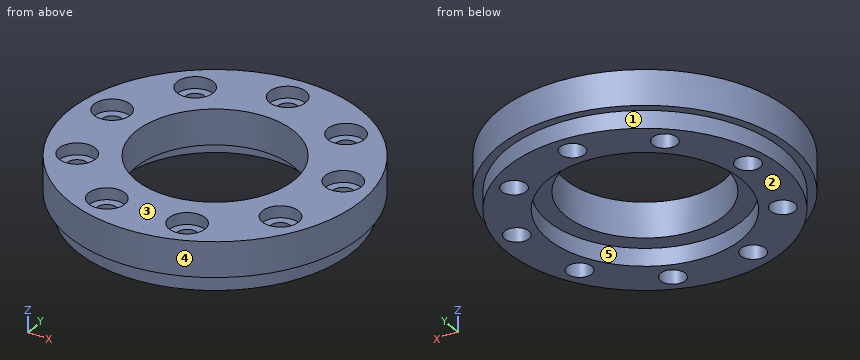
```python
from build123d import *

# Parameters (mm, degrees)
ESQUISSE1_R             = 24.95
BOSS_EXTRU_1_DEPTH      = 6
ESQUISSE3_R             = 3.1
ENL_V_MAT_EXTRU_1_DEPTH = 2
ESQUISSE4_R             = 1.7
ENL_V_MAT_EXTRU_2_DEPTH = 7
ESQUISSE5_R             = 23.5
ESQUISSE5_R_2           = 16.5
ESQUISSE5_R_3           = 1.7
BOSS_EXTRU_2_DEPTH      = 3
ESQUISSE6_R             = 2.1
ENL_V_MAT_EXTRU_3_DEPTH = 5.7
ESQUISSE7_R             = 13.5
ENL_V_MAT_EXTRU_4_DEPTH = 7


with BuildPart() as part:
    # Esquisse1 → Boss.-Extru.1 (new body)
    with BuildSketch(Plane.XY):
        Circle(ESQUISSE1_R)
    extrude(amount=BOSS_EXTRU_1_DEPTH)

    # Esquisse3 → Enlèv. mat.-Extru.1 (cut)
    with BuildSketch(Plane(origin=(0, 0, 6), x_dir=(-1, 0, 0), z_dir=(0, 0, -1))):
        with Locations((0, 20)):
            Circle(ESQUISSE3_R)
        with Locations((12.855752194, 15.320888862)):
            Circle(ESQUISSE3_R)
        with Locations((19.69615506, 3.472963553)):
            Circle(ESQUISSE3_R)
        with Locations((17.320508076, -10)):
            Circle(ESQUISSE3_R)
        with Locations((6.840402867, -18.793852416)):
            Circle(ESQUISSE3_R)
        with Locations((-6.840402867, -18.793852416)):
            Circle(ESQUISSE3_R)
        with Locations((-17.320508076, -10)):
            Circle(ESQUISSE3_R)
        with Locations((-19.69615506, 3.472963553)):
            Circle(ESQUISSE3_R)
        with Locations((-12.855752194, 15.320888862)):
            Circle(ESQUISSE3_R)
    extrude(amount=ENL_V_MAT_EXTRU_1_DEPTH, mode=Mode.SUBTRACT)

    # Esquisse4 → Enlèv. mat.-Extru.2 (cut, through all)
    with BuildSketch(Plane(origin=(0, 0, 0), x_dir=(-1, 0, 0), z_dir=(0, 0, -1))):
        with Locations((0, 20)):
            Circle(ESQUISSE4_R)
        with Locations((12.855752194, 15.320888862)):
            Circle(ESQUISSE4_R)
        with Locations((19.69615506, 3.472963553)):
            Circle(ESQUISSE4_R)
        with Locations((17.320508076, -10)):
            Circle(ESQUISSE4_R)
        with Locations((6.840402867, -18.793852416)):
            Circle(ESQUISSE4_R)
        with Locations((-6.840402867, -18.793852416)):
            Circle(ESQUISSE4_R)
        with Locations((-17.320508076, -10)):
            Circle(ESQUISSE4_R)
        with Locations((-19.69615506, 3.472963553)):
            Circle(ESQUISSE4_R)
        with Locations((-12.855752194, 15.320888862)):
            Circle(ESQUISSE4_R)
    extrude(amount=-ENL_V_MAT_EXTRU_2_DEPTH, mode=Mode.SUBTRACT)

    # Esquisse5 → Boss.-Extru.2 (add)
    with BuildSketch(Plane(origin=(0, 0, 0), x_dir=(-1, 0, 0), z_dir=(0, 0, -1))):
        Circle(ESQUISSE5_R)
        Circle(ESQUISSE5_R_2, mode=Mode.SUBTRACT)
        with Locations((-12.855752194, 15.320888862)):
            Circle(ESQUISSE5_R_3, mode=Mode.SUBTRACT)
        with Locations((-19.69615506, 3.472963553)):
            Circle(ESQUISSE5_R_3, mode=Mode.SUBTRACT)
        with Locations((-17.320508076, -10)):
            Circle(ESQUISSE5_R_3, mode=Mode.SUBTRACT)
        with Locations((-6.840402867, -18.793852416)):
            Circle(ESQUISSE5_R_3, mode=Mode.SUBTRACT)
        with Locations((6.840402867, -18.793852416)):
            Circle(ESQUISSE5_R_3, mode=Mode.SUBTRACT)
        with Locations((17.320508076, -10)):
            Circle(ESQUISSE5_R_3, mode=Mode.SUBTRACT)
        with Locations((19.69615506, 3.472963553)):
            Circle(ESQUISSE5_R_3, mode=Mode.SUBTRACT)
        with Locations((12.855752194, 15.320888862)):
            Circle(ESQUISSE5_R_3, mode=Mode.SUBTRACT)
        with Locations((0, 20)):
            Circle(ESQUISSE5_R_3, mode=Mode.SUBTRACT)
    extrude(amount=BOSS_EXTRU_2_DEPTH)

    # Esquisse6 → Enlèv. mat.-Extru.3 (cut)
    with BuildSketch(Plane(origin=(0, 0, -3), x_dir=(-1, 0, 0), z_dir=(0, 0, -1))):
        with Locations((12.855752194, 15.320888862)):
            Circle(ESQUISSE6_R)
        with Locations((19.69615506, 3.472963553)):
            Circle(ESQUISSE6_R)
        with Locations((17.320508076, -10)):
            Circle(ESQUISSE6_R)
        with Locations((6.840402867, -18.793852416)):
            Circle(ESQUISSE6_R)
        with Locations((-6.840402867, -18.793852416)):
            Circle(ESQUISSE6_R)
        with Locations((-17.320508076, -10)):
            Circle(ESQUISSE6_R)
        with Locations((-19.69615506, 3.472963553)):
            Circle(ESQUISSE6_R)
        with Locations((-12.855752194, 15.320888862)):
            Circle(ESQUISSE6_R)
        with Locations((0, 20)):
            Circle(ESQUISSE6_R)
    extrude(amount=-ENL_V_MAT_EXTRU_3_DEPTH, mode=Mode.SUBTRACT)

    # Esquisse7 → Enlèv. mat.-Extru.4 (cut, through all)
    with BuildSketch(Plane(origin=(0, 0, 0), x_dir=(-1, 0, 0), z_dir=(0, 0, -1))):
        Circle(ESQUISSE7_R)
    extrude(amount=-ENL_V_MAT_EXTRU_4_DEPTH, mode=Mode.SUBTRACT)


solid = part.part
```
Verification items for the finished model (mm, model axes). Face numbers are marked on the shaded views. A direction names the side the tool comes from. Coordinates: 2 decimals unless noted, no trailing zeros. Loops run counter-clockwise (first coordinate to the right, second up) from the corner with the lowest first, then second, coordinate; pieces in that order, holes last. Notation, with made-up numbers: (61.25, -38) - (97.25, -38) arc R27 ccw to (97.25, -16) - close; hole circle Ø10 at (48, 54.25). An arc over 180 degrees is marked (long way). Answer as a JSON object with one key per item and string values.
(1) Cross-section at B-B, the plane y = 20. Record the boundary of the cut face in (x, z).
Response:
{"outline": "(-14.92, 0) - (-12.34, 0) - (-12.34, -3) - (-2.1, -3) - (-2.1, 2.7) - (-1.7, 2.7) - (-1.7, 4) - (-3.1, 4) - (-3.1, 6) - (-14.92, 6) - close; (1.7, 2.7) - (2.1, 2.7) - (2.1, -3) - (12.34, -3) - (12.34, 0) - (14.92, 0) - (14.92, 6) - (3.1, 6) - (3.1, 4) - (1.7, 4) - close"}
(2) Go/stop test with flat-tipped pins: pin 1 Ø3 at (y, z) = (10.5, 2.5) entering from +X; pin 2 Ø7 at (x, y) = (-12.86, 15.32) entering from -Z; pin 3 Ø16.5 at (x, y) = (-0.5, 5.5) entering from -Z; pin 4 Ø1.9 at (x, y) = (14, 16.5) entering from +Z. Record where each tip stops, or that it passes through.
Response:
{"pin 1": "stops at x = 23.27", "pin 2": "stops at z = -3", "pin 3": "stops at z = 0", "pin 4": "stops at z = 4"}
(3) Cross-section at A-A, the plane x = 0. Record the boundary of the cut face in (y, z), then the cut area to 3 significant figures.
Response:
{"outline": "(-24.95, 0) - (-23.5, 0) - (-23.5, -3) - (-16.5, -3) - (-16.5, 0) - (-13.5, 0) - (-13.5, 6) - (-24.95, 6) - close; (13.5, 0) - (16.5, 0) - (16.5, -3) - (17.9, -3) - (17.9, 2.7) - (18.3, 2.7) - (18.3, 4) - (16.9, 4) - (16.9, 6) - (13.5, 6) - close; (21.7, 2.7) - (22.1, 2.7) - (22.1, -3) - (23.5, -3) - (23.5, 0) - (24.95, 0) - (24.95, 6) - (23.1, 6) - (23.1, 4) - (21.7, 4) - close", "area": "139 mm²"}
(4) Scan lines: line 1 along Y through (x, z) = (0, 5.5); line 2 along Y through (x, z) = (0, -2.25); line 3 along X through (y, z) = (-8.5, -1.75). Record each from-to range of solid material in increasing order.
Response:
{"line 1": "y = -24.95 to -13.5, 13.5 to 16.9, 23.1 to 24.95", "line 2": "y = -23.5 to -16.5, 16.5 to 17.9, 22.1 to 23.5", "line 3": "x = -21.91 to -18.79, -15.85 to -14.14, 14.14 to 15.85, 18.79 to 21.91"}
(5) Cross-section at D-D, the plane x = 7. Record the boundary of the cut face in (y, z).
Response:
{"outline": "(-23.95, 0) - (-22.43, 0) - (-22.43, -3) - (-20.89, -3) - (-20.89, 2.7) - (-20.49, 2.7) - (-20.49, 4) - (-21.89, 4) - (-21.89, 6) - (-23.95, 6) - close; (-17.1, 2.7) - (-16.7, 2.7) - (-16.7, -3) - (-14.94, -3) - (-14.94, 0) - (-11.54, 0) - (-11.54, 6) - (-15.7, 6) - (-15.7, 4) - (-17.1, 4) - close; (11.54, 0) - (14.94, 0) - (14.94, -3) - (22.43, -3) - (22.43, 0) - (23.95, 0) - (23.95, 6) - (11.54, 6) - close"}
(6) Mould release check, pull along Y, two halves, no side actions. Record for the marked faces 3, 4 and 5: pulls with the +Y half, pulls with the -Y half, needs draft (parallel to the pull), parting line crosses it, or undercut.
Response:
{"face 3": "needs draft", "face 4": "parting line crosses it", "face 5": "undercut"}
(7) Access from +Z, -Z, +X, -X, +Y, -Y to the whole of each face (thin tool, end or side, straight path). Record for the marked faces 1 and 2.
Response:
{"face 1": "-Z", "face 2": "-Z, +X, -X, +Y, -Y"}
(8) Cross-section at C-C, the plane z = -1.25. Count the separate pieces of the cut face and the enclosed holes in it, then the cut area to 3 significant figures.
Response:
{"separate pieces": "1", "enclosed holes": "10", "area": "755 mm²"}
